Verification items for the finished model (mm, model axes). Face numbers are marked on the shaded views. Round coordinates to 2 decimals unless told otherwise and drop trailing zeros. Loops run counter-clockwise (first coordinate to the right, second up) from the corner with the lowest first, then second, coordinate; pieces in that order, holes last. Notation, with made-up numbers: M 22.5,-23.75 L 74.5,-23.75 A10 cw 74.5,-18.75 Z; hole C 89.25,-28 d5. An arc over 180 degrees is marked long. Write item = value, one per line. Start each with the question number.
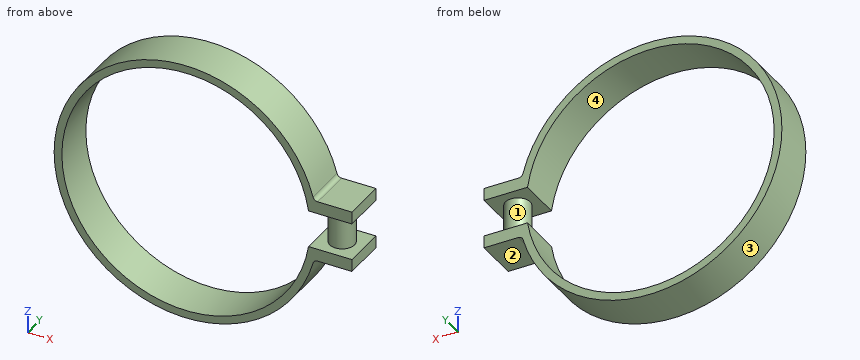
from build123d import *

# Parameters (mm, degrees)
BOSS_EXTRUDE1_DEPTH = 4.445
BOSS_EXTRUDE2_REACH = 32.797
SKETCH2_R           = 2.54


with BuildPart() as part:
    # Sketch1 → Boss-Extrude1 (new body, symmetric)
    with BuildSketch(Plane(origin=(0, 0, 0), x_dir=(1, 0, 0), z_dir=(0, 1, 0))):
        with BuildLine():
            Line((34.002624315, 3.81), (25.112624315, 3.81))
            ThreePointArc((25.112624315, 3.81), (-25.4, 0), (25.112624315, -3.81))
            Line((25.112624315, -3.81), (34.002624315, -3.81))
            Line((34.002624315, -3.81), (34.002624315, -6.35))
            Line((34.002624315, -6.35), (26.9875, -6.35))
            ThreePointArc((26.9875, -6.35), (26.394067972, -6.550896579), (26.04470524, -7.070960699))
            ThreePointArc((26.04470524, -7.070960699), (-26.9875, 0), (26.04470524, 7.070960699))
            ThreePointArc((26.04470524, 7.070960699), (26.394067972, 6.550896579), (26.9875, 6.35))
            Line((26.9875, 6.35), (34.002624315, 6.35))
            Line((34.002624315, 6.35), (34.002624315, 3.81))
        make_face()
    extrude(amount=BOSS_EXTRUDE1_DEPTH, both=True)

    # Sketch2 → Boss-Extrude2 (add, up to next)
    with BuildSketch(Plane.XY.offset(-3.81), mode=Mode.PRIVATE) as boss_extrude2_sk1:
        with Locations((29.557624315, 0)):
            Circle(SKETCH2_R)
    boss_extrude2_tool1 = extrude(boss_extrude2_sk1.sketch, amount=BOSS_EXTRUDE2_REACH, mode=Mode.PRIVATE) - part.part
    add(boss_extrude2_tool1.solids().sort_by_distance((29.557624, 0, -3.81))[0])


solid = part.part
1. Section check A-A, the plane x = 0. Enter the section's corners in (y, z) (1 decimal), and give its area (3 significant figures).
2. Gauge pin test, flat ends, axial feed: P1, Ø2, axis at y = -1, z = -16, coming from the +X side; P2, Ø5, axis at x = -1.5, y = -1.5, coming from the -Z side; P3, Ø2, axis at x = 29.5, y = -0.5, coming from the +Z side. Record the tip position at first contact, or that the pin passes through.
3. Section check B-B, the plane z = 0. Enter the section's corners in (x, y) (1 decimal), and give its area (3 significant figures).
4. Mould release check, pull along Z, two halves, no side actions. Record for the marked faces 1, 2, 3 and 4: pulls with the +Z half, pulls with the -Z half, needs draft (parallel to the pull), parting line crosses it, or undercut.
5. Thickness scan on line 1 (Z direction, x = 0, y = 0.75); line 2 (X direction, y = -2, z = -5.5); line 3 (X direction, y = -0.25, z = 17). Record the ranges inside material, lowest first.
Computed values:
q1.outline = M -4.4,-27 L 4.4,-27 L 4.4,-25.4 L -4.4,-25.4 Z; M -4.4,25.4 L 4.4,25.4 L 4.4,27 L -4.4,27 Z
q1.area = 28.2 mm2
q2.P1 = 22.43
q2.P2 = -26.99
q2.P3 = 6.35
q3.outline = M -27,-4.4 L -25.4,-4.4 L -25.4,4.4 L -27,4.4 Z; C 29.6,0 d5.1
q3.area = 34.4 mm2
q4.face_1 = undercut
q4.face_2 = pulls with the -Z half
q4.face_3 = parting line crosses it
q4.face_4 = undercut
q5.line_1 = -26.99 to -25.4, 25.4 to 26.99
q5.line_2 = -26.42 to -24.8, 24.8 to 34
q5.line_3 = -20.96 to -18.87, 18.87 to 20.96
